Geometry: final body of the model. Coordinates: model frame, mm. A direction names the side the tool comes from. Give positions to 0.01 mm unless a question says otherwise; leave off trailing zeros. Loops run counter-clockwise (first coordinate to the right, second up) from the corner with the lowest first, then second, coordinate; pieces in that order, holes last. Notation, with made-up numbers: M 30.5,67.5 L 60.5,67.5 A11 cw 60.5,83.5 Z; hole C 12.25,68 d4. An arc over 180 degrees is marked long. Put each result on its own line as item: value.
```python
from build123d import *

# Parameters (mm, degrees)
SKETCH1_W               = 110
SKETCH1_H               = 90
BOSS_EXTRUDE1_DEPTH     = 3
SKETCH2_W               = 110
SKETCH2_H               = 90
SKETCH2_W_2             = 106
SKETCH2_H_2             = 86
BOSS_EXTRUDE2_DEPTH     = 35
SKETCH3_R               = 3
BOSS_EXTRUDE3_DEPTH     = 3
SKETCH4_R               = 1.5
CUT_EXTRUDE1_DEPTH      = 78.935871074
CUT_EXTRUDE2_DEPTH      = 2.3
CUT_EXTRUDE3_REACH      = 114.112
SKETCH6_W               = 9
SKETCH6_H               = 3.5
SKETCH6_W_2             = 14
SKETCH6_H_2             = 13
SKETCH6_H_3             = 7
FILLET2_R               = 2
SKETCH7_W               = 7
SKETCH7_H               = 7
BOSS_EXTRUDE4_DEPTH     = 6
CUT_EXTRUDE4_DEPTH      = 2.2
SKETCH10_R              = 1.5
CUT_EXTRUDE5_DEPTH      = 5
CHAMFER2_SIZE           = 7
MIRROR4_COPY_1_SKETCH_W = 7
MIRROR4_COPY_1_SKETCH_H = 7
MIRROR4_COPY_1_DEPTH    = 6
MIRROR4_COPY_2_DEPTH    = 2.2
MIRROR4_COPY_3_SKETCH_R = 1.5
MIRROR4_COPY_3_DEPTH    = 5
CHAMFER3_SIZE           = 7
CHAMFER4_SIZE           = 7
FILLET6_R               = 2
CHAMFER5_SIZE           = 1.5


with BuildPart() as part:
    # Sketch1 → Boss-Extrude1 (new body)
    with BuildSketch(Plane(origin=(0, 0, 0), x_dir=(1, 0, 0), z_dir=(0, 1, 0))):
        Rectangle(SKETCH1_W, SKETCH1_H)
    extrude(amount=BOSS_EXTRUDE1_DEPTH)

    # Sketch2 → Boss-Extrude2 (add)
    with BuildSketch(Plane(origin=(0, 3, 0), x_dir=(1, 0, 0), z_dir=(0, 1, 0))):
        Rectangle(SKETCH2_W, SKETCH2_H)
        Rectangle(SKETCH2_W_2, SKETCH2_H_2, mode=Mode.SUBTRACT)
    extrude(amount=BOSS_EXTRUDE2_DEPTH)

    # Sketch3 → Boss-Extrude3 (add)
    with BuildSketch(Plane(origin=(0, 3, 0), x_dir=(1, 0, 0), z_dir=(0, 1, 0))):
        with Locations(Location((-46, 33, 0), (0, 0, 270))):
            Circle(SKETCH3_R)
        with Locations(Location((40, 33, 0), (0, 0, 270))):
            Circle(SKETCH3_R)
        with Locations(Location((-46, -25, 0), (0, 0, 270))):
            Circle(SKETCH3_R)
        with Locations(Location((40, -25, 0), (0, 0, 270))):
            Circle(SKETCH3_R)
    extrude(amount=BOSS_EXTRUDE3_DEPTH)

    # Sketch4 → Cut-Extrude1 (cut, through all)
    with BuildSketch(Plane(origin=(0, 6, 0), x_dir=(1, 0, 0), z_dir=(0, 1, 0))):
        with Locations(Location((-46, 33, 0), (0, 0, 270))):
            Circle(SKETCH4_R)
        with Locations(Location((40, 33, 0), (0, 0, 270))):
            Circle(SKETCH4_R)
        with Locations(Location((40, -25, 0), (0, 0, 270))):
            Circle(SKETCH4_R)
        with Locations(Location((-46, -25, 0), (0, 0, 270))):
            Circle(SKETCH4_R)
    extrude(amount=-CUT_EXTRUDE1_DEPTH, mode=Mode.SUBTRACT)

    # Sketch5 → Cut-Extrude2 (cut)
    with BuildSketch(Plane.XZ):
        Polygon((37.45, 26.472243186), (37.45, 23.527756814), (40, 22.055513627), (42.55, 23.527756814), (42.55, 26.472243186), (40, 27.944486373), align=None)
        Polygon((-46, 27.944486373), (-48.55, 26.472243186), (-48.55, 23.527756814), (-46, 22.055513627), (-43.45, 23.527756814), (-43.45, 26.472243186), align=None)
        Polygon((-48.55, -34.472243186), (-46, -35.944486373), (-43.45, -34.472243186), (-43.45, -31.527756814), (-46, -30.055513627), (-48.55, -31.527756814), align=None)
        Polygon((42.55, -34.472243186), (42.55, -31.527756814), (40, -30.055513627), (37.45, -31.527756814), (37.45, -34.472243186), (40, -35.944486373), align=None)
    extrude(amount=-CUT_EXTRUDE2_DEPTH, mode=Mode.SUBTRACT)

    # Sketch6 → Cut-Extrude3 (cut, up to next)
    with BuildSketch(Plane.XY.offset(45), mode=Mode.PRIVATE) as cut_extrude3_sk1:
        with Locations((-43.919999919, 9.236200323)):
            Rectangle(SKETCH6_W, SKETCH6_H)
    cut_extrude3_tool1 = extrude(cut_extrude3_sk1.sketch, amount=-CUT_EXTRUDE3_REACH, mode=Mode.PRIVATE) & part.part
    # Sketch6 → Cut-Extrude3 (cut, up to next)
    with BuildSketch(Plane.XY.offset(45), mode=Mode.PRIVATE) as cut_extrude3_sk2:
        with Locations((26.950000009, 13.355009857)):
            Rectangle(SKETCH6_W_2, SKETCH6_H_2)
    cut_extrude3_tool2 = extrude(cut_extrude3_sk2.sketch, amount=-CUT_EXTRUDE3_REACH, mode=Mode.PRIVATE) & part.part
    # Sketch6 → Cut-Extrude3 (cut, up to next)
    with BuildSketch(Plane.XY.offset(45), mode=Mode.PRIVATE) as cut_extrude3_sk3:
        with Locations((-7.4, 11.595)):
            Rectangle(SKETCH6_W_2, SKETCH6_H_3)
    cut_extrude3_tool3 = extrude(cut_extrude3_sk3.sketch, amount=-CUT_EXTRUDE3_REACH, mode=Mode.PRIVATE) & part.part
    add(cut_extrude3_tool1.solids().sort_by_distance((-43.92, 9.2362, 45))[0], mode=Mode.SUBTRACT)
    add(cut_extrude3_tool2.solids().sort_by_distance((26.95, 13.35501, 45))[0], mode=Mode.SUBTRACT)
    add(cut_extrude3_tool3.solids().sort_by_distance((-7.4, 11.595, 45))[0], mode=Mode.SUBTRACT)

    # Fillet2
    fillet2_edges = [part.edges().sort_by_distance(p)[0] for p in [
        (0, 0, 45),
        (-55, 0, 0),
        (0, 0, -45),
        (55, 0, 0),
        (55, 19, 45),
        (-55, 19, 45),
        (-55, 19, -45),
        (55, 19, -45),
    ]]
    fillet(fillet2_edges, radius=FILLET2_R)

    # Sketch7 → Boss-Extrude4 (add)
    with BuildSketch(Plane(origin=(0, 36, 0), x_dir=(1, 0, 0), z_dir=(0, 1, 0))):
        with Locations((-49.5, 39.5)):
            Rectangle(SKETCH7_W, SKETCH7_H)
    boss_extrude4 = extrude(amount=-BOSS_EXTRUDE4_DEPTH)

    # Sketch8 → Cut-Extrude4 (cut)
    with BuildSketch(Plane(origin=(0, 34, 0), x_dir=(1, 0, 0), z_dir=(0, 1, 0))):
        Polygon((-48.527756814, 42.55), (-51.472243186, 42.55), (-52.944486373, 40), (-51.472243186, 37.45), (-48.527756814, 37.45), (-46, 37.45), (-46, 42.55), align=None)
    cut_extrude4 = extrude(amount=-CUT_EXTRUDE4_DEPTH, mode=Mode.SUBTRACT)

    # Sketch10 → Cut-Extrude5 (cut)
    with BuildSketch(Plane(origin=(0, 36, 0), x_dir=(1, 0, 0), z_dir=(0, 1, 0))):
        with Locations(Location((-50, 40, 0), (0, 0, 270))):
            Circle(SKETCH10_R)
    cut_extrude5 = extrude(amount=-CUT_EXTRUDE5_DEPTH, mode=Mode.SUBTRACT)

    # Chamfer2
    chamfer2_edges = [part.edges().sort_by_distance(p)[0] for p in [
        (-53, 30, -39.5),
    ]]
    chamfer(chamfer2_edges, length=CHAMFER2_SIZE - 0.0001)  # a hair under: the kernel refuses the full size

    # Mirror3: Boss-Extrude4, Cut-Extrude4, Cut-Extrude5 across plane
    add(boss_extrude4.mirror(Plane(origin=(0, 0, 0), x_dir=(0, 0, 1), z_dir=(1, 0, 0))))
    add(cut_extrude4.mirror(Plane(origin=(0, 0, 0), x_dir=(0, 0, 1), z_dir=(1, 0, 0))), mode=Mode.SUBTRACT)
    add(cut_extrude5.mirror(Plane(origin=(0, 0, 0), x_dir=(0, 0, 1), z_dir=(1, 0, 0))), mode=Mode.SUBTRACT)

    # Mirror4: Boss-Extrude4, Cut-Extrude4, Cut-Extrude5 across plane
    add(boss_extrude4.mirror(Plane.XY))
    add(cut_extrude4.mirror(Plane.XY), mode=Mode.SUBTRACT)
    add(cut_extrude5.mirror(Plane.XY), mode=Mode.SUBTRACT)

    # Mirror4 copy 1 sketch → Mirror4 copy 1 (add)
    with BuildSketch(Plane(origin=(0, 36, 0), x_dir=(-1, 0, 0), z_dir=(0, 1, 0))):
        with Locations((-49.5, 39.5)):
            Rectangle(MIRROR4_COPY_1_SKETCH_W, MIRROR4_COPY_1_SKETCH_H)
    extrude(amount=-MIRROR4_COPY_1_DEPTH)

    # Mirror4 copy 2 sketch → Mirror4 copy 2 (cut)
    with BuildSketch(Plane(origin=(0, 34, 0), x_dir=(-1, 0, 0), z_dir=(0, 1, 0))):
        Polygon((-48.527756814, 42.55), (-51.472243186, 42.55), (-52.944486373, 40), (-51.472243186, 37.45), (-48.527756814, 37.45), (-46, 37.45), (-46, 42.55), align=None)
    extrude(amount=-MIRROR4_COPY_2_DEPTH, mode=Mode.SUBTRACT)

    # Mirror4 copy 3 sketch → Mirror4 copy 3 (cut)
    with BuildSketch(Plane(origin=(0, 36, 0), x_dir=(-1, 0, 0), z_dir=(0, 1, 0))):
        with Locations(Location((-50, 40, 0), (0, 0, 270))):
            Circle(MIRROR4_COPY_3_SKETCH_R)
    extrude(amount=-MIRROR4_COPY_3_DEPTH, mode=Mode.SUBTRACT)

    # Chamfer3
    chamfer3_edges = [part.edges().sort_by_distance(p)[0] for p in [
        (53, 30, -39.5),
    ]]
    chamfer(chamfer3_edges, length=CHAMFER3_SIZE - 0.0001)  # a hair under: the kernel refuses the full size

    # Chamfer4
    chamfer4_edges = [part.edges().sort_by_distance(p)[0] for p in [
        (-53, 30, 39.5),
        (53, 30, 39.5),
    ]]
    chamfer(chamfer4_edges, length=CHAMFER4_SIZE - 0.0001)  # a hair under: the kernel refuses the full size

    # Fillet6
    fillet6_edges = [part.edges().sort_by_distance(p)[0] for p in [
        (-53, 13.00005, -43),
        (53, 13.00005, -43),
        (-53, 13.00005, 43),
        (53, 13.00005, 43),
    ]]
    fillet(fillet6_edges, radius=FILLET6_R)

    # Chamfer5
    chamfer5_edges = [part.edges().sort_by_distance(p)[0] for p in [
        (-46, 3, -36),
        (40, 3, -36),
        (40, 3, 22),
        (-46, 3, 22),
    ]]
    chamfer(chamfer5_edges, length=CHAMFER5_SIZE)


solid = part.part
```
Item 1: Pin query (flat end, axial travel): pin 1 Ø3.5 at (x, z) = (-50.5, -39.5) entering from +Y; pin 2 Ø1.6 at (x, z) = (24, 44) entering from -Y; pin 3 Ø2.5 at (x, z) = (-46, 24.5) entering from -Y. Return the tip coordinate at first contact, or that it passes through.
Output values:
pin 1: y = 36
pin 2: y = 0.01
pin 3: y = 2.3
Item 2: Section B-B on x = 8. Output: boundary loops of the cut face in (y, z), then the cut area to 3 significant figures.
Output values:
outline: M 0,-43 A2 ccw 2,-45 L 38,-45 L 38,-43 L 3,-43 L 3,43 L 38,43 L 38,45 L 2,45 A2 ccw 0,43 Z
area: 408 mm²
Item 3: Line query: probe 1 along Z at (x, y) = (50, 35); probe 2 along X at (y, z) = (35.4, -40); probe 3 along X at (y, z) = (30.5, -26.5). Output: solid intervals per line, ascending. Write a range as [from, to].
Output values:
probe 1: [-45, -41.5], [-38.5, -36], [36, 38.5], [41.5, 45]
probe 2: [-55, -51.5], [-48.5, -46], [46, 48.5], [51.5, 55]
probe 3: [-55, -53], [53, 55]
Item 4: Section C-C on z = 25. Count the separate pieces of the cut face and the enclosed holes in it, then the cut area to 3 significant figures.
Output values:
separate pieces: 3
enclosed holes: 0
area: 463 mm²
Item 5: Set-up query: faces 4 (the flat face through (46, 34.4, -39.5)), 5 (the flat face through (-43.45, 1, 25)), 6 (the flat face through (-48, 34, 40)). Return all of +Z, -Z, +X, -X, +Y, -Y with unobstructed straight access to the full face (end or side cutting, diameter ignored); none if empty.
Output values:
face 4: +Y
face 5: -Y
face 6: none
Item 6: Mould query, pull axis X, two halves, no side actions, for faces 1 (the flat face through (55, 20, 1)), 2 (the flat face through (53, 20, 1)), 3 (the flat face through (-1, 20, 45)). Classes: pulls with the +X half, pulls with the -X half, needs draft (parallel to the pull), parting line crosses it, or undercut.
Output values:
face 1: pulls with the +X half
face 2: undercut
face 3: needs draft
Item 7: Section A-A on z = -0.5. Output: boundary loops of the cut face in (x, y).
Output values:
outline: M -55,2 A2 ccw -53,0 L 53,0 A2 ccw 55,2 L 55,38 L 53,38 L 53,3 L -53,3 L -53,38 L -55,38 Z
